For this review, use the dimensioned drawing (mm, ordinates from the lowest corner) and the shaded views. A direction names the side the tool comes from. Coordinates: 2 decimals unless noted, no trailing zeros. Loops run counter-clockwise (first coordinate to the right, second up) from the corner with the lowest first, then second, coordinate; pieces in that order, holes last. Notation, with made-up numbers: M 17.5,-9.5 L 66.5,-9.5 A20 ccw 66.5,-0.5 Z; hole C 21.25,-38 d4. An arc over 180 degrees is marked long. Write item = value, one per line. Start each with the question number.
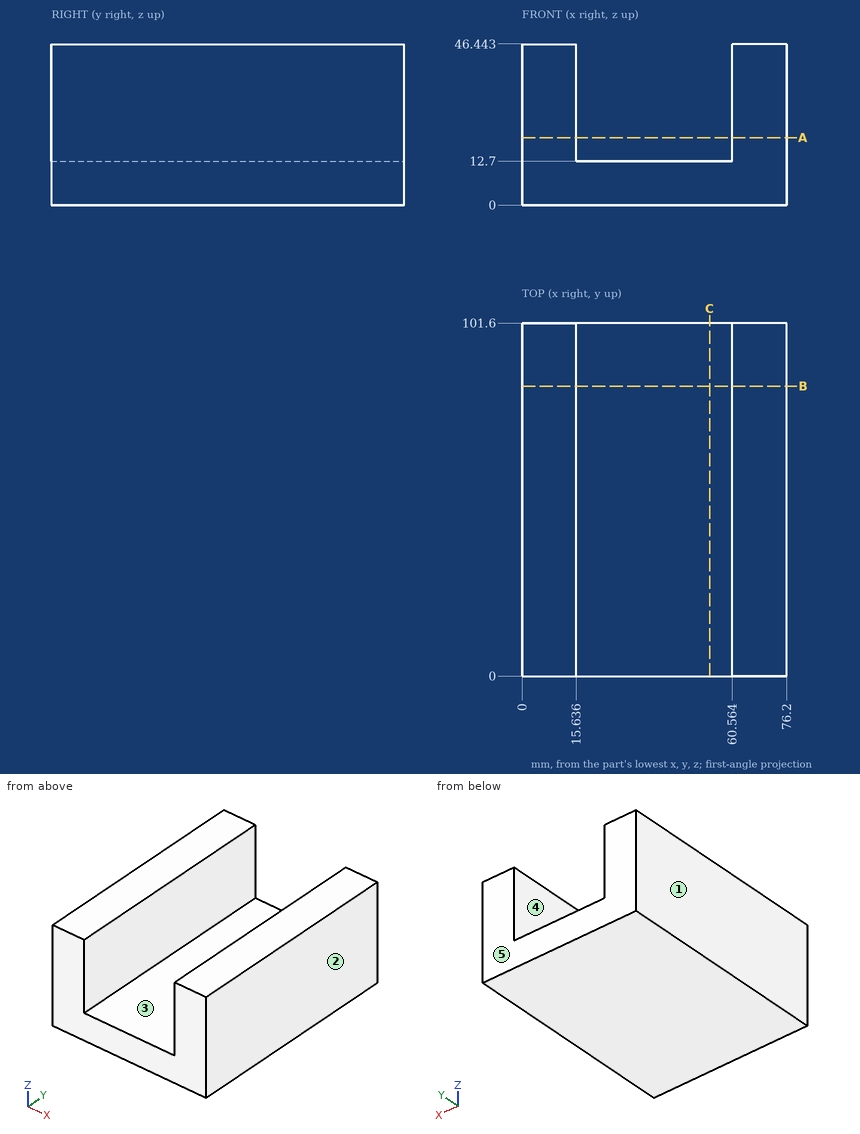
Q1. Add section A-A on z = 19.5. State the section outline as (x, y) points, plus the area to 3 significant figures.
Q2. Mouldability with a two-part tool opening along X and no side actions: class the marked faces 1, 2 and 3 as released by +X, released by -X, zero draft, split by the parting line, or undercut.
Q3. Clearance check with a flat-ended pin moving along its axis: P1, Ø22.5, axis at x = 28, y = 41, coming from the +Z side. State where the tip first meets the part, or that it passes through.
Q4. For the marked faces 4 and 5, list the 3-axis set-ups (+Z, -Z, +X, -X, +Y, -Y) from which the entire face can be reached by the end or side of a thin tool; tool diameter is ignored.
Q5. To check wall thickness, follow line 1 (X direction, y = 8.5, z = 42); line 2 (Z direction, x = 35, y = 50). State the ranges of each line that lie inside material, in increasing order. Write a range as from..to.
Q6. Add section B-B on y = 83.5. State the section outline as (x, z) points.
Q7. Add section C-C on x = 54. State the section outline as (y, z) points, plus the area to 3 significant figures.
Values follow:
q1.outline = M 0,0 L 15.64,0 L 15.64,101.6 L 0,101.6 Z; M 60.56,0 L 76.2,0 L 76.2,101.6 L 60.56,101.6 Z
q1.area = 3,180 mm2
q2.face_1 = released by -X
q2.face_2 = released by +X
q2.face_3 = undercut
q3.P1 = 12.7
q4.face_4 = +Z, +Y, -Y
q4.face_5 = +Z, -Z, +X, -X, +Y
q5.line_1 = 0..15.64, 60.56..76.2
q5.line_2 = 0..12.7
q6.outline = M 0,0 L 76.2,0 L 76.2,46.44 L 60.56,46.44 L 60.56,12.7 L 15.64,12.7 L 15.64,46.44 L 0,46.44 Z
q7.outline = M 0,0 L 101.6,0 L 101.6,12.7 L 0,12.7 Z
q7.area = 1,290 mm2
